Could you check a few things on this model? Use its own coordinates, in mm. A direction names the side the tool comes from. Give positions to 0.01 mm unless a question says otherwise; leave off trailing zeros. Order: outer loops, then holes, each group sorted by start corner. A loop starts at its lowest first (then second) coordinate and runs counter-clockwise, first axis right, second up.
from build123d import *

# Parameters (mm, degrees)
PAD_DEPTH       = 20
POCKET_DEPTH    = 3.5
POCKET001_DEPTH = 3.5
SKETCH004_R     = 6
POCKET002_DEPTH = 16.501


with BuildPart() as part:
    # Sketch001 → Pad (new body)
    with BuildSketch(Plane.XY):
        Polygon((-16.5, 20), (16.5, 20), (28, 0), (10, 0), (10, -150), (-10, -150), (-10, 0), (-28, 0), align=None)
    extrude(amount=PAD_DEPTH)

    # Sketch002 (on Face10 of Pad) → Pocket (cut)
    with BuildSketch(Plane.XY.offset(20)):
        Polygon((28, 0), (-8.68, 0), (-8.68, 20), (16.5, 20), align=None)
    extrude(amount=-POCKET_DEPTH, mode=Mode.SUBTRACT)

    # Sketch003 (on Face2 of Pocket) → Pocket001 (cut)
    with BuildSketch(Plane(origin=(0, 0, 0), x_dir=(1, 0, 0), z_dir=(0, 0, -1))):
        Polygon((28, 0), (-8.68, 0), (-8.68, -20), (16.5, -20), align=None)
    extrude(amount=-POCKET001_DEPTH, mode=Mode.SUBTRACT)

    # Sketch004 (on Face6 of Pocket001) → Pocket002 (cut, through all)
    with BuildSketch(Plane.XY.offset(16.5)):
        with Locations((1.32, 10)):
            Circle(SKETCH004_R)
    extrude(amount=-POCKET002_DEPTH, mode=Mode.SUBTRACT)


solid = part.part
Item 1: Imagine slicing it at A-A on z = 8. List the corners of the cut face in (x, y) for me, then the cut area to 3 significant figures.
Findings:
outline: (-28, 0) - (-10, 0) - (-10, -150) - (10, -150) - (10, 0) - (28, 0) - (16.5, 20) - (-16.5, 20) - close; hole circle Ø12 at (1.32, 10)
area: 3,780 mm2
Item 2: Imagine slicing it at D-D on x = 21.5. List the corners of the cut face in (y, z) for me.
Findings:
outline: (0, 3.5) - (11.3, 3.5) - (11.3, 16.5) - (0, 16.5) - close
Item 3: Imagine slicing it at B-B on y = 10. List the corners of the cut face in (x, z) for me, then the cut area to 3 significant figures.
Findings:
outline: (-22.25, 0) - (-8.68, 0) - (-8.68, 3.5) - (-4.68, 3.5) - (-4.68, 16.5) - (-8.68, 16.5) - (-8.68, 20) - (-22.25, 20) - close; (7.32, 3.5) - (22.25, 3.5) - (22.25, 16.5) - (7.32, 16.5) - close
area: 517 mm2
Item 4: We'd pull the mould along X, two halves only. Please class faces 1 (the flat face through (9, 10, 3.5)), 2 (the flat face through (-10, -76, 10)), 3 (the flat face through (22.17, 10.14, 9.91)), 4 (the cylindrical face through (0.019, 4.143, 10.091)): +X half, -X half, draft (parallel to the pull), parting line (faces both ways), or undercut.
Findings:
face 1: draft
face 2: -X half
face 3: +X half
face 4: undercut
Item 5: For pin 1 (6 mm diameter, centred on y = -46, z = 6.5, fed in from -X); pin 2 (4 mm diameter, centred on x = 23.5, z = 13, fed in from -Y); pin 3 (3 mm diameter, centred on x = 1, z = 18.5, fed in from +Y), each with a flat end and sliding along its axis, tell me the tip position at first contact or that it passes through.
Findings:
pin 1: stops at x = -10
pin 2: stops at y = 0
pin 3: stops at y = 0
Item 6: Imagine slicing it at C-C on x = 1.5. List the corners of the cut face in (y, z) for me, then the cut area to 3 significant figures.
Findings:
outline: (-150, 0) - (0, 0) - (0, 3.5) - (4, 3.5) - (4, 16.5) - (0, 16.5) - (0, 20) - (-150, 20) - close; (16, 3.5) - (20, 3.5) - (20, 16.5) - (16, 16.5) - close
area: 3,100 mm2
Item 7: Please list where these lines run through material, in increasing order: line 1 along Y through (x, z) = (1.32, 7.25); line 2 along X through (y, z) = (-91, 16); line 3 along Z through (x, y) = (20, 10).
Findings:
line 1: y = -150 to 4, 16 to 20
line 2: x = -10 to 10
line 3: z = 3.5 to 16.5
Item 8: For faces 5 (the flat face through (1, 0, 2)), 6 (the flat face through (19, 0, 10)), 7 (the flat face through (-8.68, 10, 18)), which set-ups out of +Z, -Z, +X, -X, +Y, -Y let a thin tool reach every point of the face, with its end or its side?
Findings:
face 5: -Z, +X, +Y
face 6: +Z, -Z, +X, -Y
face 7: +Z, +X, +Y
